Autodesk Inventor part; units mm, degrees
ref_plane "YZ Plane" through (0, 0, 0) normal (1, 0, 0) x (0, 1, 0)
ref_plane "XZ Plane" through (0, 0, 0) normal (0, 1, 0) x (-1, 0, 0)
ref_plane "XY Plane" through (0, 0, 0) normal (0, 0, 1) x (1, 0, 0)
sketch "Эскиз1" plane through (0, 0, 0) normal (0, 1, 0) x (-1, 0, 0)
  line L0 (40, 22) -> (0, 22)
  line L1 (0, 22) -> (0, 0)
  line L2 (0, 0) -> (40, 0)
  line L3 (40, 0) -> (40, 22)
  circle A0 centre (33.9283, 18.2892) radius 2
  circle A1 centre (33.9283, 3.7108) radius 2
  circle A2 centre (9.8763, 18.4209) radius 2
  circle A3 centre (9.8763, 3.5791) radius 2
  dimension "d0" = 40
  dimension "d1" = 22
  dimension "d2" = 4
  dimension "d3" = 4
  dimension "d4" = 4
  dimension "d5" = 4
  dimension "d6" = 6.0717
  dimension "d7" = 6.0717
  dimension "d8" = 3.7108
  dimension "d9" = 3.7108
  dimension "d10" = 9.8763
  dimension "d11" = 9.8763
  dimension "d12" = 3.5791
  dimension "d13" = 3.5791
extrude "Выдавливание1" add sketch "Эскиз1" along normal blind 4
fillet "Сопряжение1" radius 2 12 edges at (0, 2, 22) (0, 2, 0) (-40, 2, 0) (-40, 2, 22) (-40, 0, 11) (-40, 4, 11) (-20, 0, 22) (-20, 4, 22) (0, 0, 11) (0, 4, 11) (-20, 0, 0) (-20, 4, 0)
The listing builds one solid part. Answer for the finished solid, in the listing's coordinates (mm). A direction names the side the tool comes from. Give positions to 0.01 mm unless a question says otherwise; leave off trailing zeros. Answer in a Markdown table with one row per item. Add a question column.
Q1. Given P1, Ø1.5, axis at y = 1, z = 11, coming from the +X side, flat-ended and moving along its own axis, determine where the tip first touches the part or whether it passes through.
Q2. Which of the six approach directions +Z, -Z, +X, -X, +Y, -Y give full straight-line access (tool end or side, diameter ignored) to faces 4 (the cylindrical face through (-5.37, 3.43, 0.6)), 5 (the cylindrical face through (-5.37, 0.6, 0.57)), 6 (the cylindrical face through (-36.5, 0.6, 0.57))?
Q3. For a pull along Z with two mould halves and no side action, classify faces 1 (the cylindrical face through (-22.15, 0.6, 0.57)), 2 (the cylindrical face through (-0.57, 0.6, 10.87)), 3 (the cylindrical face through (-7.88, 1.97, 3.49)) as released by +Z, released by -Z, zero draft, split by the parting line, or undercut.
Q4. Find the intervals of material crossed by line 1 along Z through (x, y) = (-34, 2.05); line 2 along X through (y, z) = (0.7, 2.75); line 3 along X through (y, z) = (2.55, 17.25), in increasing order. Write a range as [from, to].
Q5. The part is cut by section B-B (z = 4.5). Give the number of separate pieces and of enclosed holes in the cut face, then the cut area to 3 significant figures.
Determined:
| question | item | result |
|---|---|---|
| 1 | P1 | stops at x = -0.02 |
| 2 | face 4 | -Z, +X, +Y |
| 2 | face 5 | -Z, +X, -Y |
| 2 | face 6 | -Z, -X, -Y |
| 3 | face 1 | released by -Z |
| 3 | face 2 | zero draft |
| 3 | face 3 | undercut |
| 4 | line 1 | z = [0, 1.71], [5.71, 16.29], [20.29, 22] |
| 4 | line 2 | x = [-39.52, -35.68], [-32.17, -11.7], [-8.06, -0.48] |
| 4 | line 3 | x = [-39.92, -35.64], [-32.22, -11.5], [-8.25, -0.08] |
| 5 | separate pieces | 3 |
| 5 | enclosed holes | 0 |
| 5 | area | 128 mm² |
